Work out the finished part from the listing and answer in its coordinate system (mm). A direction names the side the tool comes from. Give positions to 0.01 mm unless a question says otherwise; leave off trailing zeros. Loops run counter-clockwise (first coordinate to the right, second up) from the corner with the lowest first, then second, coordinate; pieces in that order, holes last. Notation, with made-up numbers: (53, 11.5) -> (108, 11.5) arc R30 cw to (108, 50.5) -> close; hole circle Ø10 at (-21, 48.25). An arc over 180 degrees is marked (long way). Answer as CSV lines item,"result". Start each with the question number.
1. Find section A-A, the plane z = 0. Give the vertices of the cut face in (x, y), and give its area (3 significant figures).
2. Find section D-D, the plane x = -20. Give the vertices of the cut face in (y, z), and give its area (3 significant figures).
3. A tool of negligible diameter and unlimited length cuts with its end or side. For faces 1 (the face through (204, 50, -1)), 2 (the face through (430, 25, 0)), from which of +Z, -Z, +X, -X, +Y, -Y can it reach the whole face along a straight path? Write none if from no direction.
4. Find section B-B, the plane y = 15.5. Give the vertices of the cut face in (x, z).
5. Find the intervals of material crossed by line 1 along X through (y, z) = (8, -3); line 2 along X through (y, z) = (6.5, -18); line 3 along X through (y, z) = (46, 43), in increasing order.
6. Flat-ended cylindrical pins translate along their axes: pin 1 Ø25 at (x, y) = (414, 22.5) entering from +Z (3 decimals); pin 2 Ø25 at (y, z) = (14, -2.5) entering from +X; pin 3 Ø15 at (y, z) = (13, -14.5) entering from -X. Find the tip coordinate at first contact, or state that the pin passes through.
7. Find section C-C, the plane z = -57. Give the vertices of the cut face in (x, y), and give its area (3 significant figures).
from build123d import *

# Parameters (mm, degrees)
SKETCH_1_W      = 60
SKETCH_1_H      = 60
EXTRUDE_1_DEPTH = 50


with BuildPart() as part:
    # 草图1 → 凸台-拉伸1 (new body)
    with BuildSketch(Plane(origin=(0, 0, 0), x_dir=(1, 0, 0), z_dir=(0, 1, 0))):
        with BuildLine():
            Line((0, 75), (400, 75))
            ThreePointArc((400, 75), (475, 0), (400, -75))
            Line((400, -75), (0, -75))
            ThreePointArc((0, -75), (-75, 0), (0, 75))
        make_face()
        with Locations((400, 0)):
            Rectangle(SKETCH_1_W, SKETCH_1_H, mode=Mode.SUBTRACT)
    extrude(amount=EXTRUDE_1_DEPTH)


solid = part.part
Resolved:
1,outline,"(-75, 0) -> (370, 0) -> (370, 50) -> (-75, 50) -> close; (430, 0) -> (475, 0) -> (475, 50) -> (430, 50) -> close"
1,area,"24,500 mm^2"
2,outline,"(0, -72.28) -> (50, -72.28) -> (50, 72.28) -> (0, 72.28) -> close"
2,area,"7,230 mm^2"
3,face 1,"+Z, -Z, +X, -X, +Y"
3,face 2,"+Y, -Y"
4,outline,"(0, -75) -> (400, -75) arc R75 ccw to (400, 75) -> (0, 75) arc R75 ccw to start; hole (370, -30) -> (430, -30) -> (430, 30) -> (370, 30) -> close"
5,line 1,"x = -74.94 to 370, 430 to 474.94"
5,line 2,"x = -72.81 to 370, 430 to 472.81"
5,line 3,"x = -61.45 to 461.45"
6,pin 1,"stops at z = 74.985"
6,pin 2,"stops at x = 475"
6,pin 3,"stops at x = -74.67"
7,outline,"(-48.74, 0) -> (448.74, 0) -> (448.74, 50) -> (-48.74, 50) -> close"
7,area,"24,900 mm^2"
